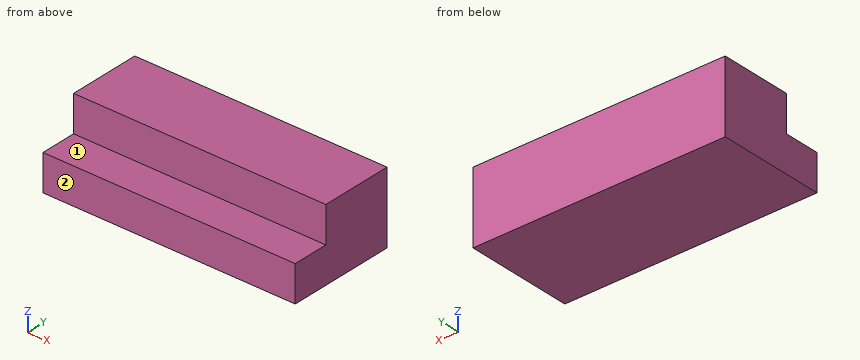
from build123d import *

# Parameters (mm, degrees)
F1_DEPTH = 25.4
F2_DEPTH = 152.4


with BuildPart() as f1:
    # F0 (on Right) → F1 (new body)
    with BuildSketch(Plane.YZ):
        Polygon((51.043449, 0), (0.243449, 0), (0.243449, -25.4), (-25.156551, -25.4), (-25.156551, -50.8), (51.043449, -50.8), align=None)
    extrude(amount=F1_DEPTH)

    # F1_face (on face) → F2 (join)
    with BuildSketch(Plane(origin=(25.4, 18.023449, -27.94), x_dir=(0, 1, 0), z_dir=(1, 0, 0))):
        Polygon((33.02, -22.86), (33.02, 27.94), (-17.78, 27.94), (-17.78, 2.54), (-43.18, 2.54), (-43.18, -22.86), align=None)
    extrude(amount=F2_DEPTH)


solid = f1.part
The model under review builds one solid part; all positions refer to its coordinate system, in mm. Face numbers are marked on the shaded views. A direction names the side the tool comes from. Give positions to 0.01 mm unless a question says otherwise; leave off trailing zeros. Loops run counter-clockwise (first coordinate to the right, second up) from the corner with the lowest first, then second, coordinate; pieces in that order, holes last. Notation, with made-up numbers: (15, -3) -> (55, -3) arc R16 cw to (55, 12) -> close; hole circle Ø6 at (31, -31.75). An arc over 180 degrees is marked (long way). Write each question's results on one line, items separated by ' | '.
1) Take a section at A-A, the plane x = 84. Give the boundary of the cut face in (y, z), plus the area to 3 significant figures.
Conclusion:
outline: (-25.16, -50.8) -> (51.04, -50.8) -> (51.04, 0) -> (0.24, 0) -> (0.24, -25.4) -> (-25.16, -25.4) -> close | area: 3,230 mm^2
2) Take a section at B-B, the plane y = -6. Give the boundary of the cut face in (x, z).
Conclusion:
outline: (0, -50.8) -> (177.8, -50.8) -> (177.8, -25.4) -> (0, -25.4) -> close
3) For line 1 along Y through (x, z) = (155, -13.5); line 2 along Z through (x, y) = (15.5, -4.5), list the stretches that pass through material, from the lowest coordinate up. Write a range as from..to.
Conclusion:
line 1: y = 0.24..51.04 | line 2: z = -50.8..-25.4
4) Insertion check: pin 1 Ø12.5 at (x, z) = (126, -10.5) entering from -Y. The pin has a flat end and moves straight along its axis. Give the tip position at first contact, or say it passes through.
Conclusion:
pin 1: stops at y = 0.24
5) Take a section at C-C, the plane z = -13.5. Give the boundary of the cut face in (x, y), plus the area to 3 significant figures.
Conclusion:
outline: (0, 0.24) -> (177.8, 0.24) -> (177.8, 51.04) -> (0, 51.04) -> close | area: 9,030 mm^2
6) Tool access review of the marked faces 1 and 2: name each direction out of +Z, -Z, +X, -X, +Y, -Y from which nothing blocks a thin tool from reaching the whole face with its end or side.
Conclusion:
face 1: +Z, +X, -X, -Y | face 2: +Z, -Z, +X, -X, -Y
